Verification items for the finished model (mm, model axes). Face numbers are marked on the shaded views. Round coordinates to 2 decimals unless told otherwise and drop trailing zeros. Write each loop counter-clockwise with the first axis right and the second up, starting at its lowest first coordinate (ties: lowest second). Pieces come first, ordered by that corner, then holes. Notation, with made-up numbers: (-33, -27.5) -> (19, -27.5) arc R31 cw to (19, 10.5) -> close; hole circle Ø6 at (35.5, 31.5). An arc over 180 degrees is marked (long way). Answer as a JSON object with one key per item and string values. Group by question number.
(1) Sectioned sample at D-D on z = 25.5. Record the cut outline in (x, y).
(2) Draft check along Y on the marked faces 1, 2 and 3. Enter one of: released by +Y, released by -Y, zero draft, split by the parting line, or undercut.
(3) Gauge pin test, flat ends, axial feed: pin 1 Ø6 at (x, y) = (55, -2) entering from +Z; pin 2 Ø0.9 at (y, z) = (44.5, 1) entering from +X; pin 3 Ø3 at (x, y) = (75, -107) entering from +Z. Record the tip position at first contact, or that the pin passes through.
(4) Sectioned sample at A-A on x = 77.5. Record the cut outline in (y, z), and give its area (3 significant figures).
(5) Scan lines: L1, parallel to Z at x = 59, y = 45; L2, parallel to X at y = 0, z = 66; L3, parallel to Y at x = 66.5, z = 77. Record each from-to range of solid material in increasing order. Write a range as from..to.
(6) Sectioned sample at C-C on y = 76.5. Record the cut outline in (x, z).
(7) Sectioned sample at B-B on z = 45.5. Record the cut outline in (x, y), and give its area (3 significant figures).
```python
from build123d import *

# Parameters (mm, degrees)
PAD_DEPTH       = 3
SKETCH001_R     = 2.5
POCKET_DEPTH    = 1.75
SKETCH002_W     = 40.796986
SKETCH002_H     = 14.7225289338
SKETCH002_R     = 2.5
POCKET001_DEPTH = 1.75
PAD001_DEPTH    = 80
SKETCH004_R     = 3.25
SKETCH004_R_2   = 1.75
POCKET002_DEPTH = 10
POCKET003_DEPTH = 10
SKETCH006_W     = 28.387858
SKETCH006_H     = 15.2811819657
POCKET004_DEPTH = 5
POCKET005_DEPTH = 1.75
SKETCH009_R     = 4
PAD002_DEPTH    = 1
POCKET006_DEPTH = 1.75
SKETCH011_R     = 4
PAD003_DEPTH    = 1


with BuildPart() as part:
    # Sketch → Pad (new body)
    with BuildSketch(Plane.XY):
        with BuildLine():
            Line((69.8529072407, 90.3022552924), (69.8529072407, -60.2396425339))
            ThreePointArc((69.8529072407, -60.2396425339), (76.0694675014, -75.2477458977), (91.0775708651, -81.4643061584))
            ThreePointArc((95.0544059368, -94.2525047463), (97.7737123274, -86.3944117953), (91.0775708651, -81.4643061584))
            Line((69.323459293, -111.9691907389), (95.0544059368, -94.2525047464))
            ThreePointArc((68.7209640656, -111.1710682539), (68.6401936472, -111.8585113494), (69.323459293, -111.9691907389))
            Line((68.7209640656, -111.1710682539), (92.8224674077, -91.2688103099))
            ThreePointArc((92.8224674077, -91.2688103099), (93.4277261515, -87.0695649029), (89.2284807399, -86.4643061907))
            Line((66.9239707498, -108.7688161808), (89.2284807722, -86.4643061584))
            ThreePointArc((49.8529072407, -101.697743289), (56.0260697472, -110.9365380783), (66.9239707498, -108.7688161808))
            Line((49.8529072407, -101.697743289), (49.8529072407, 90.3022566385))
            ThreePointArc((69.8529072407, 90.3022552924), (59.8529079137, 100.3022559338), (49.8529072407, 90.3022566385))
        make_face()
    extrude(amount=PAD_DEPTH)

    # Sketch001 → Pocket (cut)
    with BuildSketch(Plane.XY.offset(3)):
        with BuildLine():
            ThreePointArc((69.8529072407, 90.3022552924), (59.8529079137, 100.3022559338), (49.8529072407, 90.3022566385))
            Line((49.8529072407, 90.3022566385), (69.8529072407, 90.3022552924))
        make_face()
        with Locations((59.8529072407, 95.3022559338)):
            Circle(SKETCH001_R, mode=Mode.SUBTRACT)
    extrude(amount=-POCKET_DEPTH, mode=Mode.SUBTRACT)

    # Sketch002 → Pocket001 (cut)
    with BuildSketch(Plane.XY.offset(3)):
        with Locations((66.517767, -109.0590085331)):
            Rectangle(SKETCH002_W, SKETCH002_H)
        with Locations((59.8529072407, -106.6977440662)):
            Circle(SKETCH002_R, mode=Mode.SUBTRACT)
    extrude(amount=-POCKET001_DEPTH, mode=Mode.SUBTRACT)

    # Sketch007 → Pad001 (new body)
    with BuildSketch(Plane.XY.offset(3)):
        with BuildLine():
            Line((51.9742275842, 5.3629168103), (69.8529072407, -12.5157628462))
            Line((69.8529072407, -12.5157628462), (67.7315868971, -14.6370831897))
            Line((67.7315868971, -14.6370831897), (60.5600140219, -7.4655103145))
            ThreePointArc((60.5600140219, -7.4655103145), (59.8529072407, -7.1726170956), (59.1458004595, -7.4655103145))
            Line((51.9742275842, -14.6370831897), (59.1458004595, -7.4655103145))
            Line((49.8529072407, -12.5157628462), (51.9742275842, -14.6370831897))
            Line((49.8529072407, -12.5157628462), (57.0244801159, -5.3441899709))
            ThreePointArc((57.0244801159, -5.3441899709), (57.3173733348, -4.6370831897), (57.0244801159, -3.9299764085))
            Line((57.0244801159, -3.9299764085), (49.8529072407, 3.2415964667))
            Line((49.8529072407, 3.2415964667), (51.9742275842, 5.3629168103))
        make_face()
    extrude(amount=PAD001_DEPTH)

    # Sketch004 → Pocket002 (cut)
    with BuildSketch(Plane(origin=(28.6685721973, 28.6685721973, 0), x_dir=(-0.7071067812, 0.7071067812, 0), z_dir=(0.7071067812, 0.7071067812, 0))):
        with Locations((-45.601309552, 70.3578643763)):
            Circle(SKETCH004_R)
        with Locations((-39.9444553025, 64.7010101268)):
            Circle(SKETCH004_R_2)
        with Locations((-38.8837951307, 77.0753787975)):
            Circle(SKETCH004_R_2)
        with Locations((-51.2581638015, 76.0147186258)):
            Circle(SKETCH004_R_2)
        with Locations((-52.3188239733, 63.640349955)):
            Circle(SKETCH004_R_2)
        with BuildLine():
            Line((-75.5394739283, 92.3788), (-18.7021739283, 92.3788))
            Line((-18.7021739283, 92.3788), (-18.7021739283, 3))
            Line((-18.7021739283, 3), (-32.9591739283, 3))
            ThreePointArc((-34.4737045478, 64.3578643762), (-41.8644390608, 33.4778105333), (-32.9591739283, 3.0000000001))
            ThreePointArc((-34.4737045478, 64.3578643763), (-45.601309552, 83), (-56.7289145562, 64.3578643763))
            ThreePointArc((-58.2434451757, 3.0000000001), (-49.3381806572, 33.4778105485), (-56.7289145562, 64.3578643762))
            Line((-58.2434451757, 3), (-75.5394739283, 3))
            Line((-75.5394739283, 3), (-75.5394739283, 92.3788))
        make_face()
    extrude(amount=-POCKET002_DEPTH, mode=Mode.SUBTRACT)

    # Sketch005 → Pocket003 (cut)
    with BuildSketch(Plane(origin=(33.305655387, -33.305655387, 0), x_dir=(0.7071067812, 0.7071067812, 0), z_dir=(0.7071067812, -0.7071067812, 0))):
        with BuildLine():
            Line((23.5109279915, 83.5), (26.4013479915, 3))
            ThreePointArc((26.4013479915, 3.0000000001), (33.9978224249, 42.6348277252), (36.5434836152, 82.9106964523))
            Line((36.5434836152, 82.9106964523), (36.5434836152, 83.5))
            Line((36.5434836152, 83.5), (23.5109279915, 83.5))
        make_face()
    extrude(amount=-POCKET003_DEPTH, mode=Mode.SUBTRACT)

    # Sketch006 → Pocket004 (cut)
    with BuildSketch(Plane(origin=(26.5472518537, 26.5472518537, 0), x_dir=(0.7071067812, -0.7071067812, 0), z_dir=(-0.7071067812, -0.7071067812, 0))):
        with Locations((45.583672552, 77.9984553591)):
            Rectangle(SKETCH006_W, SKETCH006_H)
    extrude(amount=POCKET004_DEPTH, mode=Mode.SUBTRACT)

    # Sketch008 → Pocket005 (cut)
    with BuildSketch(Plane.XY.offset(3)):
        with BuildLine():
            Line((57.5432084738, 96.2589646702), (62.1626061364, 96.2589643593))
            ThreePointArc((62.1626061364, 96.2589643593), (59.852907409, 97.8022559338), (57.5432084738, 96.2589646702))
        make_face()
        with BuildLine():
            Line((57.543208345, 94.3455475084), (62.1626060076, 94.3455471974))
            ThreePointArc((57.543208345, 94.3455475084), (59.8529070724, 92.8022559338), (62.1626060076, 94.3455471974))
        make_face()
    extrude(amount=-POCKET005_DEPTH, mode=Mode.SUBTRACT)

    # Sketch009 → Pad002 (new body)
    with BuildSketch(Plane.XY.offset(3)):
        with Locations((59.90292, 95.269699)):
            Circle(SKETCH009_R)
    extrude(amount=PAD002_DEPTH)

    # Sketch010 → Pocket006 (cut)
    with BuildSketch(Plane.XY.offset(3)):
        with BuildLine():
            Line((57.5432084094, -105.7410354853), (62.162606072, -105.7410354853))
            ThreePointArc((62.162606072, -105.7410354853), (59.8529072407, -104.1977440662), (57.5432084094, -105.7410354853))
        make_face()
        with BuildLine():
            Line((57.5432084094, -107.6544526471), (62.162606072, -107.6544526471))
            ThreePointArc((57.5432084094, -107.6544526471), (59.8529072407, -109.1977440662), (62.162606072, -107.6544526471))
        make_face()
    extrude(amount=-POCKET006_DEPTH, mode=Mode.SUBTRACT)

    # Sketch011 → Pad003 (new body)
    with BuildSketch(Plane.XY.offset(3)):
        with Locations((59.8529072407, -106.6977440662)):
            Circle(SKETCH011_R)
    extrude(amount=PAD003_DEPTH)


solid = part.part
```
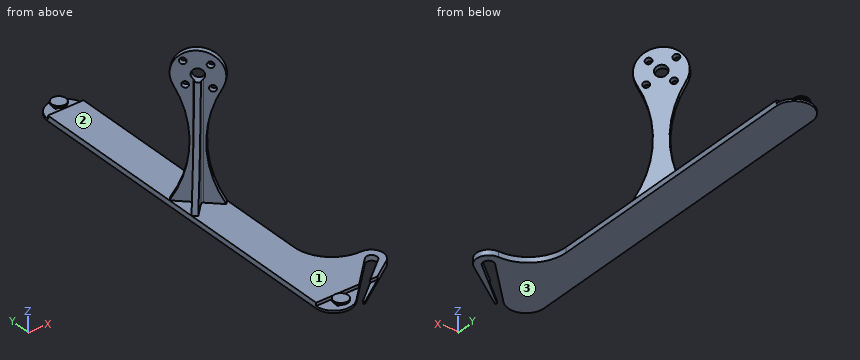
Computed values:
{
 "1": {"outline": "(53.35, -9.02) -> (55.47, -11.14) -> (59.15, -7.47) arc R1 cw to (60.56, -7.47) -> (61.94, -8.85) -> (64.06, -6.72) -> (57.77, -0.43) -> (55.64, -2.55) -> (57.02, -3.93) arc R1 cw to (57.02, -5.34) -> close"},
 "2": {"face 1": "undercut", "face 2": "undercut", "face 3": "zero draft"},
 "3": {"pin 1": "z = 82.79", "pin 2": "x = 69.85", "pin 3": "z = 1.25"},
 "4": {"outline": "(-106.34, 0) -> (-103.92, 0) -> (-103.92, 1.25) -> (-106.34, 1.25) -> close; (-98.19, 0) -> (-76.55, 0) -> (-76.55, 3) -> (-98.19, 3) -> close", "area": "67.9 mm2"},
 "5": {"L1": "0..3", "L2": "53.09..54.83", "L3": "-13.2..-9.16"},
 "6": {"outline": "(49.85, 0) -> (69.85, 0) -> (69.85, 3) -> (49.85, 3) -> close"},
 "7": {"outline": "(55.47, -6.9) -> (57.59, -9.02) -> (59.15, -7.47) arc R1 cw to (60.56, -7.47) -> (62.06, -8.96) -> (64.18, -6.84) -> (57.65, -0.31) -> (55.53, -2.43) -> (57.02, -3.93) arc R1 cw to (57.02, -5.34) -> close", "area": "37.7 mm2"}
}
